Can you work these out from the model? Positions are in its coordinate system, mm. Face numbers are marked on the shaded views. A direction names the side the tool comes from. Round coordinates to 2 decimals unless told otherwise and drop trailing zeros. Loops run counter-clockwise (first coordinate to the right, second up) from the corner with the lowest first, then second, coordinate; pieces in that order, holes last. Notation, with made-up numbers: (57.25, -19.75) -> (88.25, -19.75) arc R9 cw to (88.25, -7.75) -> close; hole circle Ø2 at (-16, 18.5). An arc over 180 degrees is marked (long way). Use a Markdown table: item, result.
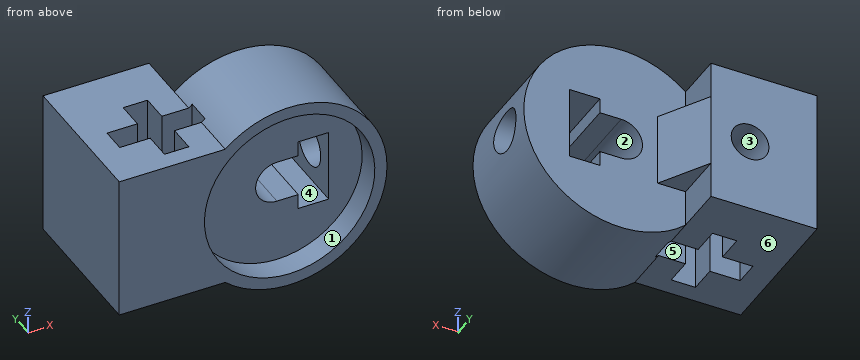
from build123d import *

# Parameters (mm, degrees)
EXTRUDE_1_DEPTH          = 8
SKETCH_4_R               = 7
CUT_EXTRUDE_3_DEPTH      = 2
SKETCH_7_W               = 8.708497378
SKETCH_7_H               = 12
EXTRUDE_2_DEPTH          = 4
SKETCH_2_R               = 1.75
CUT_EXTRUDE_1_DEPTH      = 24.260750203
CUT_EXTRUDE_2_DEPTH      = 33.695565574
CUT_EXTRUDE_2_DEPTH_BACK = 33.695565574
CUT_EXTRUDE_4_REACH      = 22.1
SKETCH_5_R               = 1.55
RIB_1_REACH              = 22.1
SKETCH_8_WALL_W          = 46.80938155
SKETCH_8_WALL_H          = 6


with BuildPart() as part:
    # 草图1 → 凸台-拉伸1 (new body)
    with BuildSketch(Plane(origin=(0, 0, 0), x_dir=(1, 0, 0), z_dir=(0, 1, 0))):
        with BuildLine():
            Line((-14, 6), (-5.291502622, 6))
            ThreePointArc((-5.291502622, 6), (8, 0), (-5.291502622, -6))
            Line((-5.291502622, -6), (-14, -6))
            Line((-14, -6), (-14, 6))
        make_face()
        with BuildLine():
            Line((1.75, 3), (1.75, 1.75))
            Line((1.75, 1.75), (0, 1.75))
            ThreePointArc((0, 1.75), (-1.75, 0), (0, -1.75))
            Line((0, -1.75), (1.75, -1.75))
            Line((1.75, -1.75), (1.75, -3))
            Line((1.75, -3), (4.25, -3))
            Line((4.25, -3), (4.25, 3))
            Line((4.25, 3), (1.75, 3))
        make_face(mode=Mode.SUBTRACT)
    extrude(amount=EXTRUDE_1_DEPTH)

    # 草图4 → 切除-拉伸3 (cut)
    with BuildSketch(Plane.XZ):
        with Locations(Location((0, 0, 0), (0, 0, 270))):
            Circle(SKETCH_4_R)
    extrude(amount=-CUT_EXTRUDE_3_DEPTH, mode=Mode.SUBTRACT)

    # 草图7 → 凸台-拉伸2 (add)
    with BuildSketch(Plane(origin=(0, 8, 0), x_dir=(1, 0, 0), z_dir=(0, 1, 0))):
        with Locations((-9.645751311, 0)):
            Rectangle(SKETCH_7_W, SKETCH_7_H)
    extrude(amount=EXTRUDE_2_DEPTH)

    # 草图2 → 切除-拉伸1 (cut, through all)
    with BuildSketch(Plane.ZY.offset(-4.25)):
        with Locations((0, 5)):
            Circle(SKETCH_2_R)
    extrude(amount=-CUT_EXTRUDE_1_DEPTH, mode=Mode.SUBTRACT)

    # 草图3 → 切除-拉伸2 (cut, two sides: drawn at the far end of the back side and taken through both)
    with BuildSketch(Plane(origin=(-19, 0, 6), x_dir=(-1, 0, 0), z_dir=(0, 0, -1)).offset(-CUT_EXTRUDE_2_DEPTH_BACK)):
        Polygon((-11.5, 1.5), (-9.5, 1.5), (-9.5, 3.75), (-7, 3.75), (-7, 5.75), (-9.5, 5.75), (-9.5, 8), (-11.5, 8), (-11.5, 5.75), (-14, 5.75), (-14, 3.75), (-11.5, 3.75), align=None)
    extrude(amount=CUT_EXTRUDE_2_DEPTH + CUT_EXTRUDE_2_DEPTH_BACK, mode=Mode.SUBTRACT)

    # 草图5 → 切除-拉伸4 (cut, up to next)
    with BuildSketch(Plane(origin=(0, 12, 0), x_dir=(1, 0, 0), z_dir=(0, 1, 0)), mode=Mode.PRIVATE) as cut_extrude_4_sk1:
        with Locations(Location((-8.5, 0, 0), (0, 0, 270))):
            Circle(SKETCH_5_R)
    cut_extrude_4_tool1 = extrude(cut_extrude_4_sk1.sketch, amount=-CUT_EXTRUDE_4_REACH, mode=Mode.PRIVATE) & part.part
    add(cut_extrude_4_tool1.solids().sort_by_distance((-8.5, 12, 0))[0], mode=Mode.SUBTRACT)

    # 草图8 wall → 筋1 (add, up to next)
    with BuildSketch(Plane(origin=(-4.145751311, 10, 0), x_dir=(0.497085200913, -0.867701736216, 0), z_dir=(0.867701736216, 0.497085200913, 0)), mode=Mode.PRIVATE) as rib_1_sk1:
        Rectangle(SKETCH_8_WALL_W, SKETCH_8_WALL_H)
    rib_1_tool1 = extrude(rib_1_sk1.sketch, amount=-RIB_1_REACH, mode=Mode.PRIVATE) - part.part
    add(rib_1_tool1.solids().sort_by_distance((-4.145751311, 10, 0))[0])


solid = part.part
1. I want a section at D-D (y = 3). Please give me the cut outline in (x, z).
Answer sheet:
| item | result |
|---|---|
| outline | (-14, -6) -> (-9.5, -6) -> (-9.5, 6) -> (-14, 6) -> close; (-7.5, -6) -> (-5.29, -6) arc R8 ccw (long way) to (-5.29, 6) -> (-7.5, 6) -> close; hole (0, -1.75) -> (1.75, -1.75) -> (1.75, -3) -> (4.25, -3) -> (4.25, 3) -> (1.75, 3) -> (1.75, 1.75) -> (0, 1.75) arc R1.75 ccw to start |
2. I need wall thicknesses on line 1 (Z direction, x = -8.5, y = 10.25); line 2 (Y direction, x = -8.25, z = -1.75); line 3 (X direction, y = 2.75, z = 1.5). Which ranges of each line are inside material? Lowest first, please.
Answer sheet:
| item | result |
|---|---|
| line 1 | z = -6 to -1.55, 1.55 to 6 |
| line 2 | y = 0 to 1.5, 8 to 12 |
| line 3 | x = -14 to -9.5, -7.5 to -0.9, 4.25 to 7.86 |
3. Will these pins go through, and if not, where does the flat tip stop? pin 1 Ø1 at (x, y) = (-5, 4) entering from +Z; pin 2 Ø1.5 at (y, z) = (11, -5) entering from +X; pin 3 Ø1.1 at (y, z) = (6.5, -4.5) entering from +X.
Answer sheet:
| item | result |
|---|---|
| pin 1 | stops at z = 6.61 |
| pin 2 | stops at x = -5.29 |
| pin 3 | stops at x = 6.96 |
4. I want a section at B-B (z = 0). State how many separate pieces and enclosed holes the cut face has, plus the area to 3 significant figures.
Answer sheet:
| item | result |
|---|---|
| separate pieces | 3 |
| enclosed holes | 0 |
| area | 100 mm² |
5. I want a section at A-A (y = 1.75). Please give me the cut outline in (x, z).
Answer sheet:
| item | result |
|---|---|
| outline | (-14, -6) -> (-9.5, -6) -> (-9.5, 6) -> (-14, 6) -> close; (-7.5, -6) -> (-5.29, -6) arc R8 ccw (long way) to (-5.29, 6) -> (-7.5, 6) -> close; hole circle Ø14 at (0, 0) |
6. If we mould it in two halves opening along Z, with no side actions, what happens to the marked faces 4, 5 and 6? For each: +Z half, -Z half, draft (parallel to the pull), parting line (faces both ways), or undercut.
Answer sheet:
| item | result |
|---|---|
| face 4 | undercut |
| face 5 | draft |
| face 6 | -Z half |
7. I want a section at C-C (x = -8.5). Please give me the cut outline in (y, z).
Answer sheet:
| item | result |
|---|---|
| outline | (0, -6) -> (1.5, -6) -> (1.5, 6) -> (0, 6) -> close; (8, -6) -> (12, -6) -> (12, -1.55) -> (8, -1.55) -> close; (8, 1.55) -> (12, 1.55) -> (12, 6) -> (8, 6) -> close |
8. Which directions (+Z, -Z, +X, -X, +Y, -Y) give clear straight access to the entire face, cutting with the end or side of a thin tool? Please do the marked faces 1, 2 and 3.
Answer sheet:
| item | result |
|---|---|
| face 1 | -Y |
| face 2 | +Y, -Y |
| face 3 | +Y |
